For this review, take the finished solid that the model builds, in its own axes (mm). Face numbers are marked on the shaded views. A direction names the side the tool comes from. Coordinates: 2 decimals unless noted, no trailing zeros. Loops run counter-clockwise (first coordinate to the right, second up) from the corner with the lowest first, then second, coordinate; pieces in that order, holes last.
1. Machinability: for the marked faces 1, 2 and 3, which of the approach directions +Z, -Z, +X, -X, +Y, -Y give a long, thin tool a straight path to every point of the face, cutting with its end or side? Answer none if there is none.
2. Mouldability with a two-part tool opening along X and no side actions: class the marked faces 4, 5, 6 and 7 as pulls with the +X half, pulls with the -X half, needs draft (parallel to the pull), parting line crosses it, or undercut.
3. Clearance check with flat-ended pins moving along their axes: P1, Ø12.5, axis at y = 28, z = -5, coming from the +X side; P2, Ø12.5, axis at x = 30.5, y = 24, coming from the +Z side; P3, Ø6, axis at x = 35, z = 18.5, coming from the +Y side. State where each tip first meets the part, or that it passes through.
4. Take a section at B-B, the plane y = 17.5. State the section outline as (x, z) points, then the cut area to 3 significant figures.
5. Take a section at D-D, the plane z = 8. State the section outline as (x, y) points.
6. Take a section at C-C, the plane x = -12. State the section outline as (y, z) points, then the cut area to 3 significant figures.
7. Take a section at A-A, the plane x = 34. State the section outline as (y, z) points, then the cut area to 3 significant figures.
8. To check wall thickness, follow probe 1 along Y at (x, z) = (-9.5, 24); probe 2 along X at (y, z) = (21.5, 29); probe 3 along Z at (x, y) = (12, 21.5). State the ranges of each line that lie inside material, in increasing order.
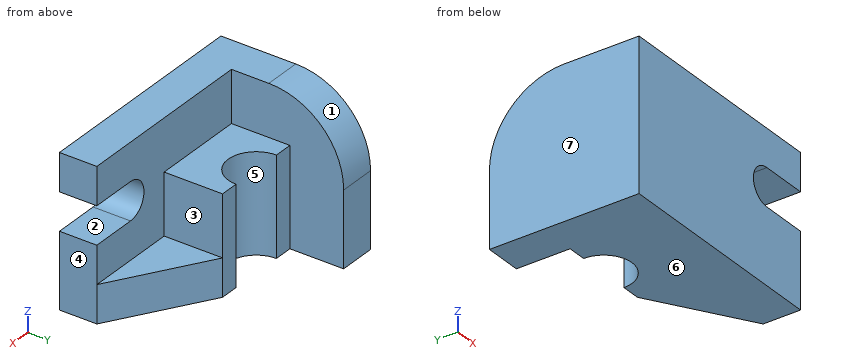
Autodesk Inventor part; units mm, degrees
ref_plane "YZ Plane" through (0, 0, 0) normal (1, 0, 0) x (0, 1, 0)
ref_plane "XZ Plane" through (0, 0, 0) normal (0, 1, 0) x (-1, 0, 0)
ref_plane "XY Plane" through (0, 0, 0) normal (0, 0, 1) x (1, 0, 0)
sketch "Sketch1" plane through (0, 0, 0) normal (0, 1, 0) x (-1, 0, 0)
  line L0 (-48, 32) -> (48, 32)
  line L1 (48, 32) -> (48, -32)
  line L2 (48, -32) -> (-48, -32)
  line L3 (-48, -32) -> (-48, 32)
  line L4 (-48, 32) -> (48, -32) construction
  line L5 (48, 32) -> (-48, -32) construction
  line L6 (-48, 16) -> (-28, 16)
  line L7 (-28, 0) -> (-48, 0)
  arc A0 (-28, 0) -> (-28, 16) centre (-28, 8) ccw
  point P0 (0, 0)
  point P1 (-38, 0)
  dimension "d0" = 96
  dimension "d1" = 64
  dimension "d3" = 16
  dimension "d4" = 16
extrude "Extrusion1" add sketch "Sketch1" along normal blind 16 contours L0 L1 L2 L3 L7 A0 L6
sketch "Sketch2" plane through (0, 16, 0) normal (0, 1, 0) x (1, 0, 0)
  line L0 (-48, 32) -> (-48, -32)
  line L1 (-48, -32) -> (48, -32)
  line L2 (-48, 32) -> (-32, 32)
  line L3 (-32, 32) -> (-32, -32)
  line L4 (-32, -32) -> (-48, -32)
  line L5 (-48, -32) -> (-48, 32)
  point P0 (0, 0)
  dimension "d8" = 16
extrude "Extrusion2" add sketch "Sketch2" along normal blind 48
fillet "Fillet1" radius 32 1 edges at (-40, 64, 32)
sketch "Sketch3" plane through (48, 0, -32) normal (0, 0, -1) x (-1, 0, 0)
  line L0 (80, 16) -> (0, 16)
  line L1 (80, 16) -> (40, 16)
  line L2 (40, 16) -> (40, 41)
  line L3 (80, 41) -> (80, 16)
  arc A0 (48, 41) -> (72, 41) centre (60, 41) ccw
  line L4 (40, 41) -> (48, 41)
  line L5 (72, 41) -> (80, 41)
  point P0 (48, 0)
  dimension "d12" = 40
  dimension "d13" = 25
extrude "Extrusion3" add sketch "Sketch3" against normal blind 42
sketch "Sketch4" plane through (48, 0, -32) normal (0, 0, -1) x (-1, 0, 0)
  line L0 (80, 16) -> (0, 16)
  line L1 (40, 41) -> (48, 41)
  line L2 (0, 16) -> (40, 41)
  line L3 (40, 16) -> (80, 16)
  line L4 (40, 41) -> (40, 16)
  line L5 (40, 16) -> (0, 16)
  point P0 (48, 0)
extrude "Extrusion4" add sketch "Sketch4" against normal blind 16
properties part number "desenho 1"
Results list:
1. face 1: +Z, +X, -X, +Y
1. face 2: +X, +Y, -Y
1. face 3: +Z, +X, +Y
2. face 4: pulls with the +X half
2. face 5: undercut
2. face 6: needs draft
2. face 7: pulls with the -X half
3. P1: stops at x = 8
3. P2: stops at z = -16
3. P3: stops at y = 16
4. outline: (-48, -32) - (45.6, -32) - (45.6, -16) - (8, -16) - (8, 10) - (-32, 10) - (-32, 32) - (-48, 32) - close
4. area: 3,310 mm2
5. outline: (-48, 0) - (20, 0) - (20, 16) - (8, 16) - (8, 41) - (0, 41) arc R12 cw to (-24, 41) - (-32, 41) - (-32, 62.98) - (-48, 62.98) - close
6. outline: (0, -32) - (29, -32) - (29, 10) - (16, 10) - (16, 32) - (0, 32) - close
6. area: 1,570 mm2
7. outline: (0, -32) - (24.75, -32) - (24.75, -16) - (16, -16) - (16, 0) - (0, 0) - close; (0, 16) - (16, 16) - (16, 32) - (0, 32) - close
7. area: 908 mm2
8. probe 1: y = 0 to 16
8. probe 2: x = -48 to -32
8. probe 3: z = -32 to -16
